from build123d import *

# Parameters (mm, degrees)
F0_W     = 40.5
F0_H     = 5
F1_DEPTH = 2
F2_W     = 5
F2_H     = 4
F3_DEPTH = 2
F4_SIZE2 = 6.99999
F4_SIZE  = 4.99999
F5_W     = 4
F5_H     = 1.25
F6_DEPTH = 2
F7_R     = 0.6
F8_DEPTH = 2


# Not quite as in the source:
# - a fillet or chamfer is up to 0.001 mm smaller than in the source, because OpenCascade refuses the exact size


with BuildPart() as f1:
    # F0 (on Front) → F1 (new body)
    with BuildSketch(Plane.XZ):
        with Locations((-20.25, 2.5)):
            Rectangle(F0_W, F0_H)
    extrude(amount=F1_DEPTH)

    # F2 (on Front) → F3 (join)
    with BuildSketch(Plane.XZ):
        with Locations((-38, -2)):
            Rectangle(F2_W, F2_H)
    extrude(amount=F3_DEPTH)

    # F4 (size 5 and 7 in the source; OpenCascade refuses exactly that, so slightly less here)
    f4_edges = [f1.edges().sort_by_distance(p)[0] for p in [
        (-40.5, -1, -4),
    ]]
    f4_side = f1.faces().sort_by_distance((-38, -1, -4))[0]
    chamfer(f4_edges, length=F4_SIZE, length2=F4_SIZE2, reference=f4_side)

    # F5 (on face) → F6 (cut)
    with BuildSketch(Plane.XZ.offset(2)):
        with Locations((-4, 2.5)):
            Rectangle(F5_W, F5_H)
    extrude(amount=-F6_DEPTH, mode=Mode.SUBTRACT)

    # F7 (on face) → F8 (cut)
    with BuildSketch(Plane.XZ.offset(2)):
        with Locations((-28.5, 2.5)):
            Circle(F7_R)
    extrude(amount=-F8_DEPTH, mode=Mode.SUBTRACT)


solid = f1.part
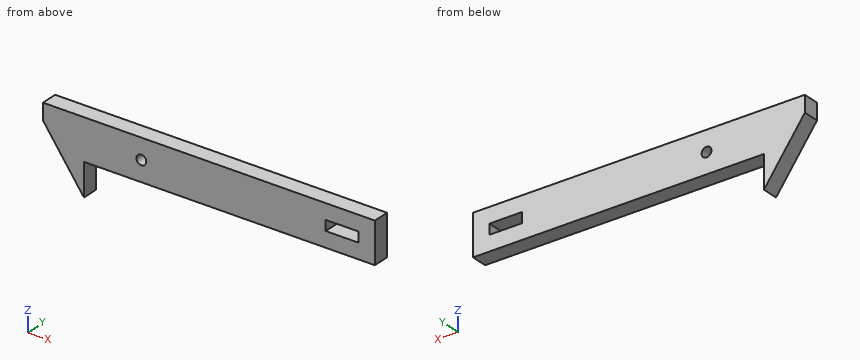
Verification items for the finished model (mm, model axes). Coordinates: 2 decimals unless noted, no trailing zeros. Write each loop counter-clockwise with the first axis right and the second up, starting at its lowest first coordinate (ties: lowest second). Pieces come first, ordered by that corner, then holes. Notation, with made-up numbers: (17.25, -5) -> (36.25, -5) arc R30 cw to (36.25, 31) -> close; hole circle Ø3 at (-31, 21.5). An arc over 180 degrees is marked (long way). One line per item, written item: value. Start each with the question number.
Q1. Cross-section at C-C on z = 2.5. Enter the section's corners in (x, y).
Q2. Cross-section at B-B on y = -0.7. State how many separate pieces and enclosed holes the cut face has, and give its area (3 significant figures).
Q3. Go/stop test with flat-tipped pins: P1, Ø0.6, axis at y = -0.5, z = -2, coming from the +X side; P2, Ø1, axis at y = -1, z = 1.5, coming from the -X side; P3, Ø1, axis at y = -1.5, z = 3, coming from the +X side. Record where each tip stops, or that it passes through.
Q4. Cross-section at A-A on x = -28.5. Enter the section's corners in (y, z), and give its area (3 significant figures).
Q5. Thickness scan on L1, parallel to Z at x = -28.5, y = -0.55; L2, parallel to Z at x = -15, y = -0.75; L3, parallel to X at y = -1.8, z = 1.75. Record the ranges inside material, lowest first. Write a range as from..to.
Q6. Cross-section at D-D on z = -0.5. Enter the section's corners in (x, y).
Checked values:
1. outline: (-40.14, -2) -> (-29.1, -2) -> (-29.1, 0) -> (-40.14, 0) -> close; (-27.9, -2) -> (-6, -2) -> (-6, 0) -> (-27.9, 0) -> close; (-2, -2) -> (0, -2) -> (0, 0) -> (-2, 0) -> close
2. separate pieces: 1
2. enclosed holes: 2
2. area: 199 mm²
3. P1: stops at x = -35.5
3. P2: stops at x = -39.79
3. P3: stops at x = 0
4. outline: (-2, 0) -> (0, 0) -> (0, 1.9) -> (-2, 1.9) -> close; (-2, 3.1) -> (0, 3.1) -> (0, 5) -> (-2, 5) -> close
4. area: 7.60 mm²
5. L1: z = 0..1.9, 3.1..5
5. L2: z = 0..5
5. L3: x = -39.61..0
6. outline: (-38, -2) -> (-35.5, -2) -> (-35.5, 0) -> (-38, 0) -> close
